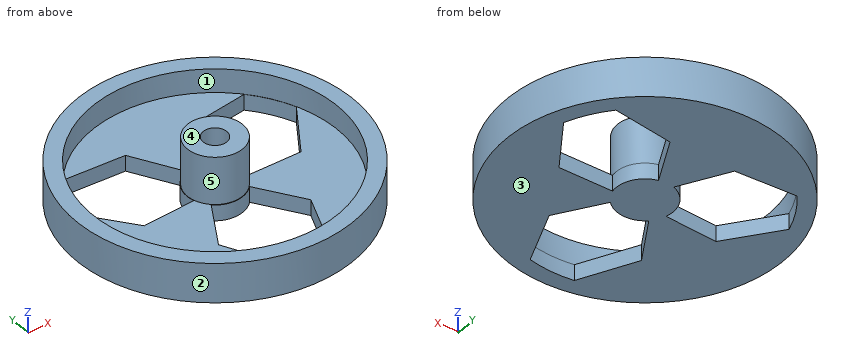
from build123d import *

# Parameters (mm, degrees)
F0_R     = 17.5
F1_DEPTH = 5
F2_R     = 15.5
F3_DEPTH = 3
F4_R     = 3.5
F4_R_2   = 1.5
F5_DEPTH = 6
F8_DEPTH = 25


with BuildPart() as f1:
    # F0 (on Top) → F1 (new body)
    with BuildSketch(Plane.XY):
        Circle(F0_R)
    extrude(amount=F1_DEPTH)

    # F2 (on face) → F3 (cut)
    with BuildSketch(Plane.XY.offset(5)):
        Circle(F2_R)
    extrude(amount=-F3_DEPTH, mode=Mode.SUBTRACT)

    # F4 (on face) → F5 (join)
    with BuildSketch(Plane.XY.offset(2)):
        Circle(F4_R)
        Circle(F4_R_2, mode=Mode.SUBTRACT)
    extrude(amount=F5_DEPTH)

    # F7 (on face) → F8 (cut)
    with BuildSketch(Plane(origin=(0, 0, 0), x_dir=(1, 0, 0), z_dir=(0, 0, -1))):
        with BuildLine():
            ThreePointArc((-2.510914, 2.59477), (0.012059, 3.554075), (2.502232, 2.512588))
            Line((2.502232, 2.512588), (6.036088, 8.101013))
            Line((6.036088, 8.101013), (2.972662, 15.185164))
            ThreePointArc((2.972662, 15.185164), (0.115894, 15.47105), (-2.744629, 15.22557))
            Line((-2.744629, 15.22557), (-6.044772, 8.347561))
            Line((-6.044772, 8.347561), (-2.510914, 2.59477))
        make_face()
        with BuildLine():
            Line((-3.427081, 0.910703), (-10.033727, 1.1769))
            Line((-10.033727, 1.1769), (-14.637069, -5.018181))
            ThreePointArc((-14.637069, -5.018181), (-13.456269, -7.635157), (-11.813416, -9.989703))
            Line((-11.813416, -9.989703), (-4.206814, -9.408706))
            Line((-4.206814, -9.408706), (-0.99168, -3.471901))
            ThreePointArc((-0.99168, -3.471901), (-3.083949, -1.766595), (-3.427081, 0.910703))
        make_face()
        with BuildLine():
            Line((0.924849, -3.423291), (3.997639, -9.277912))
            Line((3.997639, -9.277912), (11.664407, -10.166983))
            ThreePointArc((11.664407, -10.166983), (13.340375, -7.835892), (14.558044, -5.235867))
            Line((14.558044, -5.235867), (10.251585, 1.061145))
            Line((10.251585, 1.061145), (3.502594, 0.87713))
            ThreePointArc((3.502594, 0.87713), (3.07189, -1.787481), (0.924849, -3.423291))
        make_face()
    extrude(amount=-F8_DEPTH, mode=Mode.SUBTRACT)


solid = f1.part
Model file for the job. Use its own axes, mm. Face numbers are marked on the shaded views. A direction names the side the tool comes from. Give positions to 0.01 mm unless a question says otherwise; leave off trailing zeros. Order: outer loops, then holes, each group sorted by start corner. A loop starts at its lowest first (then second) coordinate and runs counter-clockwise, first axis right, second up. Notation, with made-up numbers: M 17,61.25 L 67,61.25 A12 ccw 67,70.25 Z; hole C 47,31 d5. An arc over 180 degrees is marked long. Put each result on its own line as item: value. Start each with the question number.
(1) Drill centre lines: L1, parallel to Y at x = 0, z = 3.45; L2, parallel to X at y = 7, z = 0.5; L3, parallel to Y at x = 0, z = 6. Where is each one in solid material? Low to high. Write a range as [from, to].
(2) Pull direction Y, two halves, no side cores. Call the marked faces 1, 2 and 3: released by +Y, released by -Y, zero draft, split by the parting line, or undercut.
(3) Band-saw the part on C-C on y = 7.5. Count the separate pieces of the cut face and the enclosed holes in it, then the cut area to 3 significant figures.
(4) Band-saw the part on A-A on z = 0.5. Give the cut face in (x, y).
(5) Band-saw the part on B-B on x = 7. Give the cut face in (y, z), then the cut area to 3 significant figures.
(6) Pin check, flat tips, straight feed: pin 1 Ø4 at (x, y) = (14, 2) entering from +Z; pin 2 Ø4 at (x, y) = (6.5, -0.5) entering from +Z; pin 3 Ø1.5 at (y, z) = (-12, 6) entering from +X; pin 4 Ø2 at (x, z) = (-4, 5) entering from +Y. Stop position of each tip, or through.
(7) Tool access for the marked faces 4 and 5: list every direction of +Z, -Z, +X, -X, +Y, -Y with a clear straight run to the whole face (end or side of a thin tool).
Results below:
1. L1: y = [-17.5, -15.5], [-3.5, -1.5], [1.5, 3.5], [15.5, 17.5]
1. L2: x = [-16.04, -13.8], [-2.9, 2.8], [13.8, 16.04]
1. L3: y = [-3.5, -1.5], [1.5, 3.5]
2. face 1: undercut
2. face 2: split by the parting line
2. face 3: zero draft
3. separate pieces: 3
3. enclosed holes: 0
3. area: 35.1 mm2
4. outline: C 0,0 d35; hole M -14.64,5.02 L -10.03,-1.18 L -3.43,-0.91 A3.64 cw -0.99,3.47 L -4.21,9.41 L -11.81,9.99 A15.51 ccw Z; hole M -6.04,-8.35 L -2.74,-15.23 A15.51 ccw 2.97,-15.19 L 6.04,-8.1 L 2.5,-2.51 A3.64 cw -2.51,-2.59 Z; hole M 0.92,3.42 A3.64 cw 3.5,-0.88 L 10.25,-1.06 L 14.56,5.24 A15.51 ccw 11.66,10.17 L 4,9.28 Z
5. outline: M -16.04,0 L -0.97,0 L -0.97,2 L -13.83,2 L -13.83,5 L -16.04,5 Z; M 9.63,0 L 16.04,0 L 16.04,5 L 13.83,5 L 13.83,2 L 9.63,2 Z
5. area: 56.2 mm2
6. pin 1: stops at z = 5
6. pin 2: stops at z = 2
6. pin 3: passes through
6. pin 4: stops at y = 17.24
7. face 4: +Z, +X, -X, +Y, -Y
7. face 5: +Z
